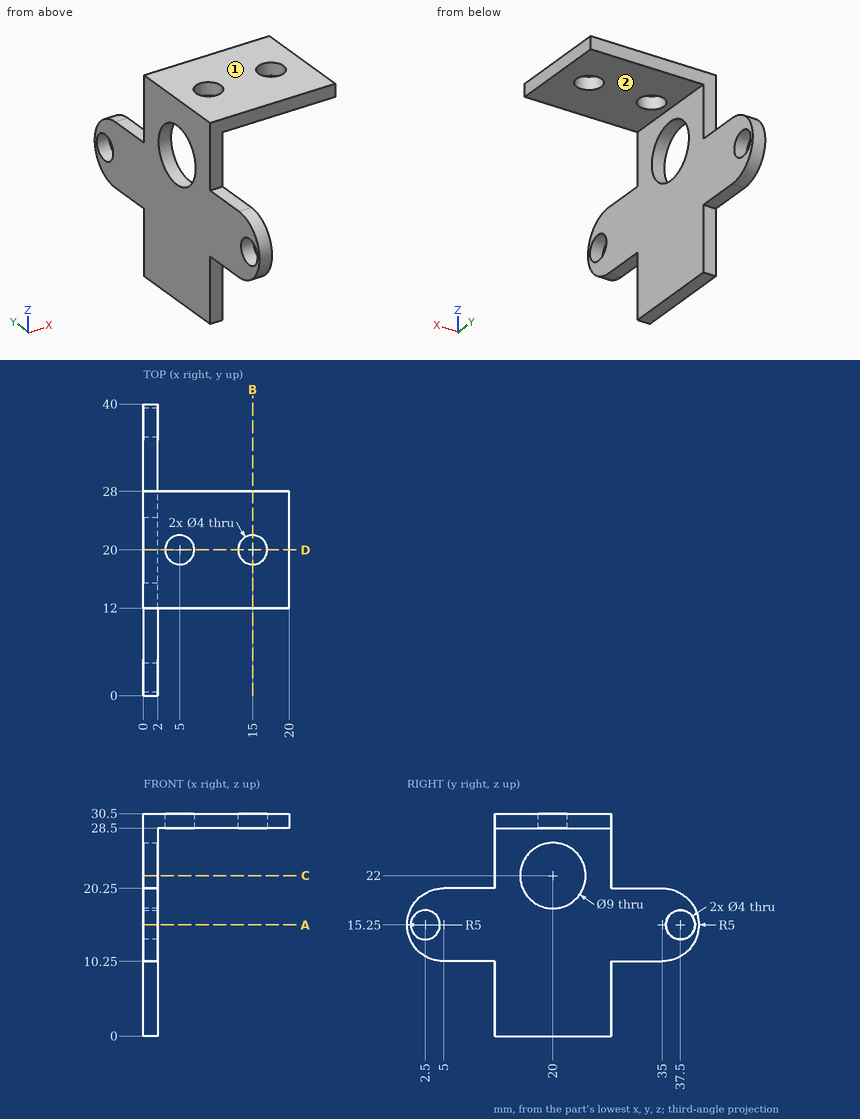
Geometry: see drawing. Coordinates: mm, zero at the bounding-box minimum. A direction names the side the tool comes from. Give positions to 0.01 mm unless a question says otherwise; leave off trailing zeros. Order: outer loops, then holes, each group sorted by start corner. A loop starts at its lowest first (then second) coordinate and runs counter-clockwise, first axis right, second up.
Q1. Section D-D on y = 20. Output: boundary loops of the cut face in (x, z), and give its area (3 significant figures).
Checked values:
outline: (0, 0) - (2, 0) - (2, 17.5) - (0, 17.5) - close; (0, 26.5) - (2, 26.5) - (2, 28.5) - (3, 28.5) - (3, 30.5) - (0, 30.5) - close; (7, 28.5) - (13, 28.5) - (13, 30.5) - (7, 30.5) - close; (17, 28.5) - (20, 28.5) - (20, 30.5) - (17, 30.5) - close
area: 63.0 mm2
Q2. Section A-A on z = 15.25. Output: boundary loops of the cut face in (x, y).
Checked values:
outline: (0, 0) - (2, 0) - (2, 0.5) - (0, 0.5) - close; (0, 4.5) - (2, 4.5) - (2, 35.5) - (0, 35.5) - close; (0, 39.5) - (2, 39.5) - (2, 40) - (0, 40) - close
Q3. Ray query, probe 1 along Y at (x, z) = (1.1, 15.25); probe 2 along Y at (x, z) = (15, 29.15); probe 3 along X at (y, z) = (27, 7). Return the intervals inside material, ascending.
Checked values:
probe 1: y = 0 to 0.5, 4.5 to 35.5, 39.5 to 40
probe 2: y = 12 to 18, 22 to 28
probe 3: x = 0 to 2
Q4. Set-up query: the marked faces 1 and 2. Return all of +Z, -Z, +X, -X, +Y, -Y with unobstructed straight access to the full face (end or side cutting, diameter ignored); none if empty.
Checked values:
face 1: +Z, +X, -X, +Y, -Y
face 2: -Z, +X, +Y, -Y
Q5. Contact query for flat-ended pins moving along their axis: pin 1 Ø8 at (x, z) = (13.5, 27) entering from -Y; pin 2 Ø3 at (y, z) = (37.5, 15.25) entering from -X; pin 3 Ø1.6 at (x, y) = (0.5, 9.5) entering from -Z; pin 4 Ø11.5 at (x, z) = (14, 24.5) entering from +Y. Output: stop coordinate, or through.
Checked values:
pin 1: stops at y = 12
pin 2: passes through
pin 3: stops at z = 10.25
pin 4: stops at y = 28
Q6. Section C-C on z = 22. Output: boundary loops of the cut face in (x, y).
Checked values:
outline: (0, 12) - (2, 12) - (2, 15.5) - (0, 15.5) - close; (0, 24.5) - (2, 24.5) - (2, 28) - (0, 28) - close
Q7. Section B-B on x = 15. Output: boundary loops of the cut face in (y, z).
Checked values:
outline: (12, 28.5) - (18, 28.5) - (18, 30.5) - (12, 30.5) - close; (22, 28.5) - (28, 28.5) - (28, 30.5) - (22, 30.5) - close
